The listing builds one solid part. Answer for the finished solid, in the listing's coordinates (mm). A direction names the side the tool comes from. Round coordinates to 2 decimals unless told otherwise and drop trailing zeros. Write each loop counter-clockwise with the first axis right and the second up, starting at its lowest first coordinate (ties: lowest second). Pieces come first, ordered by that corner, then holes. Notation, with made-up numbers: (-38.5, 71.25) - (-6.5, 71.25) arc R17 ccw to (-6.5, 88.25) - close; hole circle Ø6 at (0.5, 88.5). An arc over 180 degrees is marked (long way). Answer in a Markdown table with one row per item.
from build123d import *

# Parameters (mm, degrees)
PAD_DEPTH               = 9.65
PAD001_DEPTH            = 1.5
PAD002_DEPTH            = 1.5
SKETCH003_W             = 14.7
SKETCH003_H             = 1.07
PAD003_DEPTH            = 19
PAD004_DEPTH            = 1.1
PAD005_DEPTH            = 1.1
FILLET001_R             = 0.5
CHAMFER_SIZE            = 0.7
SKETCH011_R             = 3.75
SKETCH011_R_2           = 4.75
SKETCH011_R_3           = 5
POCKET001_DEPTH         = 5
POCKET001_DEPTH_BACK    = 5
BODY001_PLACEMENT_ANGLE = 90


with BuildPart() as part:
    # Sketch → Pad (new body, symmetric)
    with BuildSketch(Plane.YZ):
        with BuildLine():
            ThreePointArc((0, 20.5122), (-0.4209, 0), (0, -20.5122))
            ThreePointArc((0, -20.5122), (0.44097, -21.514212), (1.445369, -21.949718))
            Line((1.445369, -21.949718), (10.0791, -22.257094))
            Line((10.0791, -22.257094), (10.0791, -20.756143))
            Line((1.498737, -20.450667), (10.0791, -20.756143))
            ThreePointArc((1.498737, 20.450667), (1.0791, 0), (1.498737, -20.450667))
            Line((1.498737, 20.450667), (10.0791, 20.756143))
            Line((10.0791, 20.756143), (10.0791, 22.257094))
            Line((1.445369, 21.949718), (10.0791, 22.257094))
            ThreePointArc((1.445369, 21.949718), (0.44097, 21.514212), (0, 20.5122))
        make_face()
    extrude(amount=PAD_DEPTH, both=True)

    # Sketch001 → Pad001 (join)
    with BuildSketch(Plane.YZ.offset(9.65)):
        with BuildLine():
            ThreePointArc((0, 20.5122), (-0.4209, 0), (0, -20.5122))
            ThreePointArc((0, -20.5122), (0.44097, -21.514212), (1.445369, -21.949718))
            Line((1.445369, -21.949718), (10.0791, -22.257094))
            Line((10.0791, 22.257094), (10.0791, -22.257094))
            Line((1.445369, 21.949718), (10.0791, 22.257094))
            ThreePointArc((1.445369, 21.949718), (0.44097, 21.514212), (0, 20.5122))
        make_face()
    extrude(amount=PAD001_DEPTH)

    # Sketch002 → Pad002 (join)
    with BuildSketch(Plane.YZ.offset(-9.65)):
        with BuildLine():
            ThreePointArc((0, 20.5122), (-0.4209, 0), (0, -20.5122))
            ThreePointArc((0, -20.5122), (0.44097, -21.514212), (1.445369, -21.949718))
            Line((1.445369, -21.949718), (10.0791, -22.257094))
            Line((10.0791, 22.257094), (10.0791, -22.257094))
            Line((1.445369, 21.949718), (10.0791, 22.257094))
            ThreePointArc((1.445369, 21.949718), (0.44097, 21.514212), (0, 20.5122))
        make_face()
    extrude(amount=-PAD002_DEPTH)

    # Sketch003 → Pad003 (join)
    with BuildSketch(Plane.XZ.offset(-1)):
        with Locations((0, 20.46)):
            Rectangle(SKETCH003_W, SKETCH003_H)
        with Locations((0, -20.46)):
            Rectangle(SKETCH003_W, SKETCH003_H)
    extrude(amount=-PAD003_DEPTH)

    # Sketch004 → Pad004 (join)
    with BuildSketch(Plane.YZ.offset(7.35)):
        Polygon((1.2, 11.82), (1.2, 19.925), (20, 19.925), (20, 18.665), align=None)
        Polygon((1.2, -11.82), (1.2, -19.925), (20, -19.925), (20, -18.665), align=None)
    extrude(amount=-PAD004_DEPTH)

    # Sketch010 → Pad005 (join)
    with BuildSketch(Plane.YZ.offset(-7.35)):
        Polygon((1.2, 11.82), (1.2, 19.925), (20, 19.925), (20, 18.665), align=None)
        Polygon((1.2, -11.82), (1.2, -19.925), (20, -19.925), (20, -18.665), align=None)
    extrude(amount=PAD005_DEPTH)

    # Fillet001
    fillet001_edges = [part.edges().sort_by_distance(p)[0] for p in [
        (7.35, 10.609705, 15.246034),
        (6.25, 10.609705, 15.246034),
        (-6.25, 10.609705, 15.246034),
        (-7.35, 10.609705, 15.246034),
        (7.35, 10.609705, -15.246034),
        (6.25, 10.609705, -15.246034),
        (-6.25, 10.609705, -15.246034),
        (-7.35, 10.609705, -15.246034),
    ]]
    fillet(fillet001_edges, radius=FILLET001_R)

    # Chamfer
    chamfer_edges = [part.edges().sort_by_distance(p)[0] for p in [
        (9.65, 5.788919, 20.603405),
        (-9.65, 5.788919, 20.603405),
        (-9.65, 5.788919, -20.603405),
        (9.65, 5.788919, -20.603405),
    ]]
    chamfer(chamfer_edges, length=CHAMFER_SIZE)

    # Sketch011 → Pocket001 (cut, two sides)
    with BuildSketch(Plane.XZ) as pocket001_sk:
        Circle(SKETCH011_R)
        with Locations((0, 11)):
            Circle(SKETCH011_R_2)
        with Locations((0, -11)):
            Circle(SKETCH011_R_3)
    extrude(amount=-POCKET001_DEPTH, mode=Mode.SUBTRACT)
    extrude(pocket001_sk.sketch, amount=POCKET001_DEPTH_BACK, mode=Mode.SUBTRACT)


with BuildPart() as part_1:
    # Body001 placement: moved
    add(part.part.moved(Location((0, 0, 12))).rotate(Axis((0, 0, 12), (-1, 0, 0)), BODY001_PLACEMENT_ANGLE))


solid = part_1.part
(1) Section A-A (y = 0) is taken. Give the vertices of the cut face in (x, z), and give its area (3 significant figures).
Checked values:
| item | result |
|---|---|
| outline | (-11.15, 1.92) - (-9.65, 1.92) - (-9.65, 10.92) - (-3.75, 10.92) - (-3.75, 12.42) - (-11.15, 12.42) - close; (3.75, 10.92) - (9.65, 10.92) - (9.65, 1.92) - (11.15, 1.92) - (11.15, 12.42) - (3.75, 12.42) - close |
| area | 49.2 mm2 |
(2) Section B-B (x = 1) is taken. Give the vertices of the cut face in (y, z) (1 decimal).
Checked values:
| item | result |
|---|---|
| outline | (-22.3, 1.9) - (-21, 1.9) - (-21, -8) - (-19.9, -8) - (-19.9, 10.5) arc R498.5 cw to (-15.9, 10.7) - (-15.9, 12.2) arc R500 ccw to (-20.5, 12) arc R1.5 ccw to (-21.9, 10.6) - close; (-6.1, 10.9) arc R498.5 cw to (-3.6, 10.9) - (-3.6, 12.4) arc R500 ccw to (-6.1, 12.4) - close; (3.6, 10.9) arc R498.5 cw to (6.4, 10.9) - (6.4, 12.4) arc R500 ccw to (3.6, 12.4) - close; (15.6, 10.7) arc R498.5 cw to (19.9, 10.5) - (19.9, -8) - (21, -8) - (21, 1.9) - (22.3, 1.9) - (21.9, 10.6) arc R1.5 ccw to (20.5, 12) arc R500 ccw to (15.6, 12.2) - close |
(3) For a pull along Y with two mould halves and no side action, classify faces 3 (the flat face through (-0.1, -20.3, -8)), 4 (the flat face through (0, 20.995, -3)), 5 (the flat face through (-9.65, 0, 6)) as pulls with the +Y half, pulls with the -Y half, needs draft (parallel to the pull), parting line crosses it, or undercut.
Checked values:
| item | result |
|---|---|
| face 3 | needs draft |
| face 4 | pulls with the +Y half |
| face 5 | undercut |
(4) Flat-ended cylindrical pins translate along their axes: pin 1 (1.5 mm diameter, centred on x = 2, z = -1, fed in from +Y) (3 decimals); pin 2 (3 mm diameter, centred on x = 0, z = -4, fed in from -Y) (3 decimals); pin 3 (1 mm diameter, centred on x = 5, y = -12.5, fed in from -Z). Find the tip coordinate at first contact, or state that the pin passes through.
Checked values:
| item | result |
|---|---|
| pin 1 | stops at y = 20.995 |
| pin 2 | stops at y = -20.995 |
| pin 3 | stops at z = 10.75 |
(5) Section C-C (y = 11) is taken. Give the vertices of the cut face in (x, z).
Checked values:
| item | result |
|---|---|
| outline | (-11.15, 1.92) - (-9.65, 1.92) - (-9.65, 10.8) - (-4.75, 10.8) - (-4.75, 12.3) - (-11.15, 12.3) - close; (4.75, 10.8) - (9.65, 10.8) - (9.65, 1.92) - (11.15, 1.92) - (11.15, 12.3) - (4.75, 12.3) - close |
(6) For faces 1 (the flat face through (0, 19.925, 1)), 2 (the cylindrical face through (-0.651, -6.043, 11.537)), determine the directions among +Z, -Z, +X, -X, +Y, -Y from which every point of the face is accessible in a straight line to the end or side of a thin tool.
Checked values:
| item | result |
|---|---|
| face 1 | -Z |
| face 2 | +Z, -Z |
(7) Find the intervals of material crossed by line 1 (X direction, y = -20, z = 2); line 2 (X direction, y = -11, z = 11.7); line 3 (X direction, y = -4.5, z = 5.75), in increasing order.
Checked values:
| item | result |
|---|---|
| line 1 | x = -11.15 to -9.65, -7.35 to 7.35, 9.65 to 11.15 |
| line 2 | x = -11.15 to -5, 5 to 11.15 |
| line 3 | x = -11.15 to -9.65, 9.65 to 11.15 |
